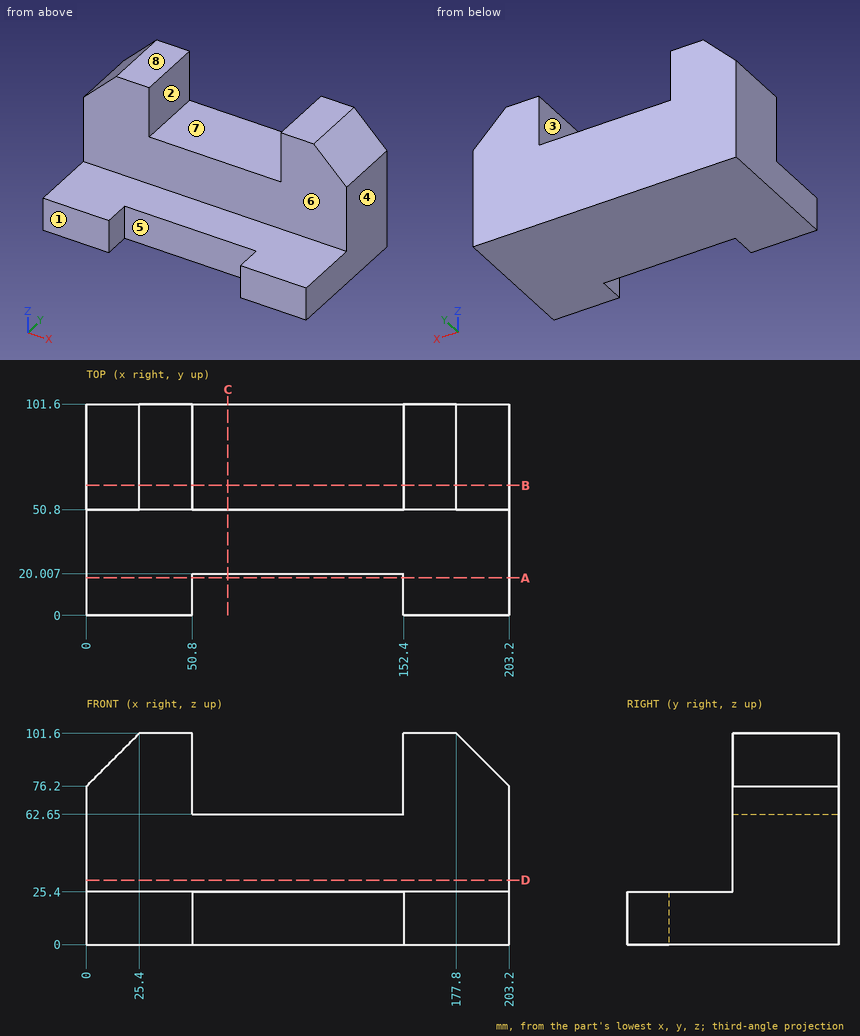
Can you work these out from the drawing? Everything is in mm from the part's minimum corner. A direction names the side the tool comes from. Give positions to 0.01 mm unless a question says otherwise; leave off trailing zeros. Loops run counter-clockwise (first coordinate to the right, second up) from the corner with the lowest first, then second, coordinate; pieces in that order, holes last. Notation, with made-up numbers: (30, 22) -> (68, 22) arc R12 ccw to (68, 33) -> close; hole circle Ø5 at (9.25, 56.5). An arc over 180 degrees is marked (long way). Write item = value, one per line.
1) Suppose I cut it at B-B on y = 62.5. Write out the boundary of the cut face in (x, z), then the cut area to 3 significant figures.
Check result:
outline = (0, 0) -> (203.2, 0) -> (203.2, 76.2) -> (177.8, 101.6) -> (152.4, 101.6) -> (152.4, 62.65) -> (50.8, 62.65) -> (50.8, 101.6) -> (25.4, 101.6) -> (0, 76.2) -> close
area = 16,000 mm2
2) For the marked faces 5, 6, 7 and 8, which set-ups out of +Z, -Z, +X, -X, +Y, -Y let a thin tool reach every point of the face, with its end or its side?
Check result:
face_5 = +Z, -Z, -Y
face_6 = +Z, +X, -X, -Y
face_7 = +Z, +Y, -Y
face_8 = +Z, +X, -X, +Y, -Y
3) Suppose I cut it at D-D on z = 31. Write out the boundary of the cut face in (x, y), then the cut area to 3 significant figures.
Check result:
outline = (0, 50.8) -> (203.2, 50.8) -> (203.2, 101.6) -> (0, 101.6) -> close
area = 10,300 mm2
4) I need wall thicknesses on L1, parallel to X at y = 76, z = 70.5; L2, parallel to Z at x = 153.5, y = 42.5; L3, parallel to Y at x = 159.5, z = 80. Which ranges of each line are inside material? Lowest first, please. Write a range as from..to.
Check result:
L1 = 0..50.8, 152.4..203.2
L2 = 0..25.4
L3 = 50.8..101.6
5) Will these pins go through, and if not, where does the flat tip stop? pin 1 (11.5 mm diameter, centred on y = 68, z = 87, fed in from +X); pin 2 (5 mm diameter, centred on x = 37, z = 66.5, fed in from -Y); pin 3 (20.5 mm diameter, centred on x = 108.5, z = 15, fed in from -Y).
Check result:
pin_1 = 198.15
pin_2 = 50.8
pin_3 = 20.01
6) Thinking about a two-plate mould opening in X: for the marked faces 1, 2, 3 and 4, which applies, released by +X, released by -X, zero draft, split by the parting line, or undercut?
Check result:
face_1 = zero draft
face_2 = undercut
face_3 = undercut
face_4 = released by +X
7) Suppose I cut it at C-C on x = 68. Write out the boundary of the cut face in (y, z), then the cut area to 3 significant figures.
Check result:
outline = (20.01, 0) -> (101.6, 0) -> (101.6, 62.65) -> (50.8, 62.65) -> (50.8, 25.4) -> (20.01, 25.4) -> close
area = 3,960 mm2
8) Suppose I cut it at A-A on y = 18. Write out the boundary of the cut face in (x, z), then the cut area to 3 significant figures.
Check result:
outline = (0, 0) -> (50.8, 0) -> (50.8, 25.4) -> (0, 25.4) -> close; (152.4, 0) -> (203.2, 0) -> (203.2, 25.4) -> (152.4, 25.4) -> close
area = 2,580 mm2
